Could you check a few things on this model? Use its own coordinates, in mm. A direction names the side the tool comes from. Coordinates: 2 decimals unless noted, no trailing zeros. Loops run counter-clockwise (first coordinate to the right, second up) from the corner with the lowest first, then second, coordinate; pieces in that order, holes last. Notation, with made-up numbers: (-13.75, 54.5) -> (38.25, 54.5) arc R32 cw to (38.25, 85.5) -> close; hole circle Ø9 at (-4.5, 1.25). An arc over 180 degrees is marked (long way). One line per question, with ' | ' between items. Start each with the question number.
(1) Which directions (+Z, -Z, +X, -X, +Y, -Y) give clear straight access to the entire face, cutting with the end or side of a thin tool? Please do faces 1 (the face through (-4.262, -0.056, -1.394)), 2 (the face through (-12.6, 0.1, 4.9)), 3 (the face through (-3, -4, 3)).
(2) Suppose I cut it at A-A (x = 2). Please give me the cut outline in (y, z).
(3) I'm going to push flat-ended pins straight in: pin 1 Ø5 at (x, z) = (8.5, 2.5) entering from +Y; pin 2 Ø2 at (y, z) = (-3.5, 5.5) entering from +X; pin 3 Ø8 at (x, z) = (-22, 4.5) entering from -Y. Where does each tip first touch, or does it pass through?
(4) If I drill on line 1 along Z through (x, y) = (20.5, 0); line 2 along X through (y, z) = (-0.5, -2); line 3 along Y through (x, z) = (-4, 6), over which ranges is the centre line in solid material (lowest first)?
(5) Suppose I cut it at D-D (x = -37.5). Please give me the cut outline in (y, z), plus the area to 3 significant figures.
(6) Suppose I cut it at C-C (x = 23). Please give me the cut outline in (y, z), plus the area to 3 significant figures.
(7) If we mould it in two halves opening along Y, with no side actions, what happens to faces 4 (the face through (-60, 0, 0)), 5 (the face through (24.93, -1.08, -4.88)), 6 (the face through (26, 0, -2))? For each: pulls with the +Y half, pulls with the -Y half, needs draft (parallel to the pull), parting line crosses it, or undercut.
```python
from build123d import *

# Parameters (mm, degrees)
F2_W           = 27
F2_H           = 10.543919
F3_DEPTH       = 12.5
F4_SIZE        = 1
F6_DEPTH       = 12.5
F8_D           = 4
F8_DEPTH       = 50
F8_CSINK_D     = 5
F8_CSINK_ANGLE = 90


with BuildPart() as f1:
    # F0 (on Top) → F1 (revolve)
    with BuildSketch(Plane.XY):
        Polygon((30.57735, 4), (30, 5), (20, 5), (13.5, 4), (10, 7.5), (0, 7.5), (-10, 7.5), (-13.5, 4), (-20, 5), (-60, 5), (-60, 0), (0, 0), (50, 0), (50, 4), align=None)
    revolve(axis=Axis((-30, 0, 0), (1, 0, 0)))

    # F2 (on Top) → F3 (cut, symmetric)
    with BuildSketch(Plane.XY):
        with Locations((0, 9.271959)):
            Rectangle(F2_W, F2_H)
        with Locations((0, -9.271959)):
            Rectangle(F2_W, F2_H)
    extrude(amount=F3_DEPTH, both=True, mode=Mode.SUBTRACT)

    # F4
    f4_edges = [f1.edges().sort_by_distance(p)[0] for p in [
        (-60, -5, 0),
        (50, -4, 0),
    ]]
    chamfer(f4_edges, length=F4_SIZE)

    # F5 (on face) → F6 (cut, symmetric)
    with BuildSketch(Plane.XZ.offset(4)):
        with BuildLine():
            ThreePointArc((-2.828427, -2.828427), (1.530734, -3.695518), (4, 0))
            ThreePointArc((4, 0), (1.530734, 3.695518), (-2.828427, 2.828427))
            ThreePointArc((-2.828427, 2.828427), (-4, 0), (-2.828427, -2.828427))
        make_face()
        with BuildLine():
            ThreePointArc((-2.828427, -2.828427), (-4, 0), (-2.828427, 2.828427))
            Line((-2.828427, 2.828427), (-5.656854, 0))
            Line((-5.656854, 0), (-2.828427, -2.828427))
        make_face()
    extrude(amount=F6_DEPTH, both=True, mode=Mode.SUBTRACT)

    # F8
    with Locations(Plane.YZ.offset(50)):
        with Locations((0, 0)):
            CounterSinkHole(F8_D / 2, F8_CSINK_D / 2, depth=F8_DEPTH, counter_sink_angle=F8_CSINK_ANGLE)


solid = f1.part
```
Checks:
1) face 1: +Y, -Y | face 2: +Z | face 3: +Z, -Z, -Y
2) outline: (-4, -6.34) arc R7.5 ccw to (4, -6.34) -> (4, -3.46) -> (-4, -3.46) -> close; (-4, 3.46) -> (4, 3.46) -> (4, 6.34) arc R7.5 ccw to (-4, 6.34) -> close
3) pin 1: stops at y = 4 | pin 2: stops at x = 11.98 | pin 3: stops at y = -4.97
4) line 1: z = -5 to -2, 2 to 5 | line 2: x = -60 to -3.66, 3.46 to 49.56 | line 3: y = -4 to 4
5) outline: circle Ø10 at (0, 0) | area: 78.5 mm^2
6) outline: circle Ø10 at (0, 0); hole circle Ø4 at (0, 0) | area: 66.0 mm^2
7) face 4: needs draft | face 5: parting line crosses it | face 6: undercut
